```python
from build123d import *

# Parameters (mm, degrees)
BOSS_EXTRUDE1_DEPTH = 7
SKETCH2_R           = 4
BOSS_EXTRUDE2_DEPTH = 8.5
SKETCH3_R           = 2.5
CUT_EXTRUDE1_DEPTH  = 10.5


with BuildPart() as part:
    # Sketch1 → Boss-Extrude1 (new body)
    with BuildSketch(Plane.XY):
        with BuildLine():
            Line((0, 0), (0, 40))
            ThreePointArc((0, 40), (-12, 52), (-24, 40))
            Line((-24, 40), (-24, 0))
            ThreePointArc((-24, 0), (-12, -12), (0, 0))
        make_face()
    extrude(amount=BOSS_EXTRUDE1_DEPTH)

    # Sketch2 → Boss-Extrude2 (add)
    with BuildSketch(Plane.XY.offset(7)):
        with Locations((-12, 0)):
            Circle(SKETCH2_R)
    extrude(amount=BOSS_EXTRUDE2_DEPTH)

    # Sketch3 → Cut-Extrude1 (cut)
    with BuildSketch(Plane.XY.offset(7)):
        with Locations((-12, 40)):
            Circle(SKETCH3_R)
    extrude(amount=-CUT_EXTRUDE1_DEPTH, mode=Mode.SUBTRACT)


solid = part.part
```
Design review of the part built by this model. Coordinates are the model's own, in mm. A direction names the side the tool comes from. Give positions to 0.01 mm unless a question says otherwise; leave off trailing zeros. Order: outer loops, then holes, each group sorted by start corner. A loop starts at its lowest first (then second) coordinate and runs counter-clockwise, first axis right, second up. Notation, with made-up numbers: (-30, 71.25) -> (-8, 71.25) arc R14 ccw to (-8, 94.25) -> close; hole circle Ø6 at (-12, -8.5). An arc over 180 degrees is marked (long way). Write item = value, one per line. Start each with the question number.
(1) We need section D-D on z = 13. Write out the cut boundary in (x, y), plus the area to 3 significant figures.
(2) We need section B-B on z = 5.75. Write out the cut boundary in (x, y).
(3) For pin 1 (3 mm diameter, centred on x = -10.5, z = 11, fed in from -Y); pin 2 (8 mm diameter, centred on x = -12, y = 40, fed in from +Z); pin 3 (2 mm diameter, centred on x = -20.5, z = 4.5, fed in from -Y); pin 4 (10 mm diameter, centred on x = -20, y = 24.5, fed in from -Z), all flat-tipped, find the tip position at first contact; note any pin that passes through.
(4) To check wall thickness, follow line 1 along Y through (x, z) = (-12, 5); line 2 along Z through (x, y) = (-3.5, 2.5); line 3 along X through (y, z) = (-0.5, 3.25). State the ranges of each line that lie inside material, in increasing order.
(5) We need section C-C on y = 7. Write out the cut boundary in (x, z).
(6) We need section A-A on x = -12. Write out the cut boundary in (y, z), plus the area to 3 significant figures.
(7) For faces 1 (the face through (-12.54, 37.56, 3.55)), 2 (the face through (-15.2, -2.4, 11.2)), list the 3-axis set-ups (+Z, -Z, +X, -X, +Y, -Y) from which the entire face can be reached by the end or side of a thin tool; tool diameter is ignored.
Numbers:
q1.outline = circle Ø8 at (-12, 0)
q1.area = 50.3 mm^2
q2.outline = (-24, 0) arc R12 ccw to (0, 0) -> (0, 40) arc R12 ccw to (-24, 40) -> close; hole circle Ø5 at (-12, 40)
q3.pin_1 = -4
q3.pin_2 = 7
q3.pin_3 = -9.37
q3.pin_4 = 0
q4.line_1 = -12 to 37.5, 42.5 to 52
q4.line_2 = 0 to 7
q4.line_3 = -23.99 to -0.01
q5.outline = (-24, 0) -> (0, 0) -> (0, 7) -> (-24, 7) -> close
q6.outline = (-12, 0) -> (37.5, 0) -> (37.5, 7) -> (4, 7) -> (4, 15.5) -> (-4, 15.5) -> (-4, 7) -> (-12, 7) -> close; (42.5, 0) -> (52, 0) -> (52, 7) -> (42.5, 7) -> close
q6.area = 481 mm^2
q7.face_1 = +Z, -Z
q7.face_2 = +Z
